Design review of the part built by this model. Coordinates are the model's own, in mm. Face numbers are marked on the shaded views. A direction names the side the tool comes from. Coordinates: 2 decimals unless noted, no trailing zeros. Order: outer loops, then holes, each group sorted by start corner. A loop starts at its lowest first (then second) coordinate and runs counter-clockwise, first axis right, second up. Notation, with made-up numbers: (-35.75, -7) -> (-21.75, -7) arc R33 cw to (-21.75, 32) -> close; hole circle Ø4 at (42, 13.25). An arc over 180 degrees is marked (long way). Write item = value, one per line.
```python
from build123d import *

# Parameters (mm, degrees)
ESBO_O2_R             = 9
CORTE_EXTRUS_O1_DEPTH = 0.1
CORTE_EXTRUS_O2_START = -0.1
ESBO_O3_R             = 9
CORTE_EXTRUS_O2_DEPTH = 0.1


with BuildPart() as part:
    # Esboço1 → Revolução1 (revolve)
    with BuildSketch(Plane(origin=(0, 0, 0), x_dir=(1, 0, 0), z_dir=(0, 1, 0))):
        with BuildLine():
            Line((9.7, -3), (6, -3))
            Line((6, -3), (6, -33))
            Line((6, -33), (9.7, -33))
            ThreePointArc((9.7, -33), (10.265685425, -32.765685425), (10.5, -32.2))
            Line((10.5, -32.2), (10.5, -29.5))
            Line((10.5, -29.5), (10, -29.5))
            Line((10, -29.5), (10, -28.2))
            Line((10, -28.2), (10.5, -28.2))
            Line((10.5, -28.2), (10.5, -7.8))
            Line((10.5, -7.8), (10, -7.8))
            Line((10, -7.8), (10, -6.5))
            Line((10, -6.5), (10.5, -6.5))
            Line((10.5, -6.5), (10.5, -3.8))
            ThreePointArc((10.5, -3.8), (10.265685425, -3.234314575), (9.7, -3))
        make_face()
    revolve(axis=Axis((0, 0, 2.998746006), (0, 0, 1)))

    # Esboço2 → Corte-extrusão1 (cut)
    with BuildSketch(Plane.XY.offset(33)):
        Circle(ESBO_O2_R)
    extrude(amount=-CORTE_EXTRUS_O1_DEPTH, mode=Mode.SUBTRACT)

    # Esboço3 → Corte-extrusão2 (cut)
    with BuildSketch(Plane(origin=(0, 0, 3), x_dir=(-1, 0, 0), z_dir=(0, 0, -1)).offset(CORTE_EXTRUS_O2_START)):
        with Locations(Location((0, 0, 0), (0, 0, 180))):
            Circle(ESBO_O3_R)
    extrude(amount=CORTE_EXTRUS_O2_DEPTH, mode=Mode.SUBTRACT)


solid = part.part
```
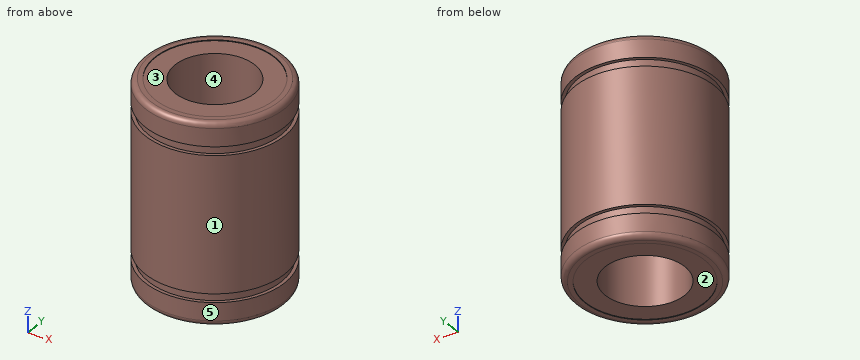
(1) For L1, parallel to Y at x = 0, z = 20.25; L2, parallel to X at y = -2, z = 31.5; L3, parallel to Y at x = 4.25, z = 24, list the stretches that pass through material, from the lowest coordinate up.
Report:
L1 = -10.5 to -6, 6 to 10.5
L2 = -10.31 to -5.66, 5.66 to 10.31
L3 = -9.6 to -4.24, 4.24 to 9.6
(2) Insertion check: pin 1 (1 mm diameter, centred on y = -2, z = 16.5, fed in from +X); pin 2 (1 mm diameter, centred on x = -3, z = 7.5, fed in from -Y); pin 3 (9.5 mm diameter, centred on x = 0, y = 0, fed in from +Z); pin 4 (6 mm diameter, centred on x = 7.5, z = 7, fed in from +Y). Each pin has a flat end and moves straight along its axis. Give the tip position at first contact, or say it passes through.
Report:
pin_1 = 10.39
pin_2 = -10.17
pin_3 = through
pin_4 = 9.47
(3) The part is to be moulded in two halves that separate along Y. For the marked faces 3, 4 and 5, say which applies: released by +Y, released by -Y, zero draft, split by the parting line, or undercut.
Report:
face_3 = undercut
face_4 = undercut
face_5 = split by the parting line
(4) For the marked faces 1 and 2, list the 3-axis set-ups (+Z, -Z, +X, -X, +Y, -Y) from which the entire face can be reached by the end or side of a thin tool; tool diameter is ignored.
Report:
face_1 = +Z, -Z
face_2 = -Z
(5) We need section A-A (z = 8.25). Write out the cut boundary in (x, y), and give its area (3 significant figures).
Report:
outline = circle Ø21 at (0, 0); hole circle Ø12 at (0, 0)
area = 233 mm²
